For this review, take the finished solid that the model builds, in its own axes (mm). A direction names the side the tool comes from. Coordinates: 2 decimals unless noted, no trailing zeros. Order: outer loops, then holes, each group sorted by start corner. A loop starts at its lowest first (then second) coordinate and runs counter-clockwise, first axis right, second up.
from build123d import *

# Parameters (mm, degrees)
BOSS_EXTRUDE2_DEPTH = 15
CUT_EXTRUDE2_REACH  = 60.655
SKETCH4_R           = 4.7625
CIRPATTERN2_COUNT   = 4


with BuildPart() as part:
    # Sketch3 → Boss-Extrude2 (new body)
    with BuildSketch(Plane(origin=(0, 0, 0), x_dir=(1, 0, 0), z_dir=(0, 1, 0))):
        Polygon((-25, -21.281601718), (25, -21.281601718), (37.466473657, -8.815128061), (37.466473657, 8.815128061), (25, 21.281601718), (-25, 21.281601718), (-37.466473657, 8.815128061), (-37.466473657, -8.815128061), align=None)
        Polygon((-34.291473657, -7.5), (-23.684871939, -18.106601718), (23.684871939, -18.106601718), (34.291473657, -7.5), (34.291473657, 7.5), (23.684871939, 18.106601718), (-23.684871939, 18.106601718), (-34.291473657, 7.5), align=None, mode=Mode.SUBTRACT)
    extrude(amount=BOSS_EXTRUDE2_DEPTH)

    # Sketch4 → Cut-Extrude2 (cut, up to next)
    with BuildSketch(Plane.XY.offset(21.281601718), mode=Mode.PRIVATE) as cut_extrude2_sk1:
        with Locations((0, 7.5)):
            Circle(SKETCH4_R)
    cut_extrude2_tool1 = extrude(cut_extrude2_sk1.sketch, amount=-CUT_EXTRUDE2_REACH, mode=Mode.PRIVATE) & part.part
    cut_extrude2 = cut_extrude2_tool1.solids().sort_by_distance((0, 7.5, 21.281602))[0]
    add(cut_extrude2, mode=Mode.SUBTRACT)

    # CirPattern2: Cut-Extrude2; each copy of Cut-Extrude2 runs up to whatever stops it at its own place
    cirpattern2_before = part.part  # the part as the pattern finds it: every copy runs up to it
    cirpattern2_cut_extrude2_long = extrude(cut_extrude2_sk1.sketch, amount=-CUT_EXTRUDE2_REACH, mode=Mode.PRIVATE)
    cirpattern2_cut_extrude2_tool1 = cirpattern2_cut_extrude2_long.rotate(Axis((0, 0, 0), (0, 1, 0)), 1 * 360 / CIRPATTERN2_COUNT) & cirpattern2_before
    add(cirpattern2_cut_extrude2_tool1.solids().sort_by_distance((21.281602, 7.5, 0))[0], mode=Mode.SUBTRACT)
    cirpattern2_cut_extrude2_tool2 = cirpattern2_cut_extrude2_long.rotate(Axis((0, 0, 0), (0, 1, 0)), 2 * 360 / CIRPATTERN2_COUNT) & cirpattern2_before
    add(cirpattern2_cut_extrude2_tool2.solids().sort_by_distance((0, 7.5, -21.281602))[0], mode=Mode.SUBTRACT)
    cirpattern2_cut_extrude2_tool3 = cirpattern2_cut_extrude2_long.rotate(Axis((0, 0, 0), (0, 1, 0)), 3 * 360 / CIRPATTERN2_COUNT) & cirpattern2_before
    add(cirpattern2_cut_extrude2_tool3.solids().sort_by_distance((-21.281602, 7.5, 0))[0], mode=Mode.SUBTRACT)


solid = part.part
1. The part is to be moulded in two halves that separate along X. For faces 3 (the face through (-37.466, 2, 0)), 4 (the face through (0, 0, -19)), 5 (the face through (28.91, 7.4, 12.88)), say which applies: +X half, -X half, draft (parallel to the pull), parting line (faces both ways), or undercut.
Answer below:
face 3: -X half
face 4: draft
face 5: undercut
2. Take a section at A-A, the plane y = 7.5. Give the number of separate pieces and of enclosed holes in the cut face, plus the area to 3 significant figures.
Answer below:
separate pieces: 4
enclosed holes: 0
area: 499 mm2
3. Take a section at D-D, the plane x = 22. Give the boundary of the cut face in (y, z).
Answer below:
outline: (0, -21.28) - (15, -21.28) - (15, -18.11) - (0, -18.11) - close; (0, 18.11) - (15, 18.11) - (15, 21.28) - (0, 21.28) - close
4. Machinability: for faces 1 (the face through (0, 2, 18.107)), 2 (the face through (-35.86, 12.22, 0.62)), which of the approach directions +Z, -Z, +X, -X, +Y, -Y give a long, thin tool a straight path to every point of the face, cutting with its end or side? Answer none if there is none.
Answer below:
face 1: +Y, -Y
face 2: +X, -X
5. Take a section at C-C, the plane x = 0. Give the boundary of the cut face in (y, z).
Answer below:
outline: (0, -21.28) - (2.74, -21.28) - (2.74, -18.11) - (0, -18.11) - close; (0, 18.11) - (2.74, 18.11) - (2.74, 21.28) - (0, 21.28) - close; (12.26, -21.28) - (15, -21.28) - (15, -18.11) - (12.26, -18.11) - close; (12.26, 18.11) - (15, 18.11) - (15, 21.28) - (12.26, 21.28) - close
6. To check wall thickness, follow L1, parallel to Z at x = -17, y = 13.5; L2, parallel to X at y = 2.75, z = 4.5; L3, parallel to Y at x = 0, z = 19.55. State the ranges of each line that lie inside material, in increasing order.
Answer below:
L1: z = -21.28 to -18.11, 18.11 to 21.28
L2: x = -37.47 to -34.29, 34.29 to 37.47
L3: y = 0 to 2.74, 12.26 to 15
7. Take a section at B-B, the plane z = -6. Give the boundary of the cut face in (x, y), plus the area to 4 significant figures.
Answer below:
outline: (-37.47, 0) - (-34.29, 0) - (-34.29, 15) - (-37.47, 15) - close; (34.29, 0) - (37.47, 0) - (37.47, 15) - (34.29, 15) - close
area: 95.25 mm2
